Can you work these out from the model? Positions are in its coordinate system, mm. A direction names the side the tool comes from. Give positions to 0.01 mm unless a question says otherwise; leave off trailing zeros. Order: outer loops, then holes, each group sorted by start corner. A loop starts at its lowest first (then second) coordinate and runs counter-clockwise, first axis right, second up.
```python
from build123d import *

# Parameters (mm, degrees)
F0_W     = 127
F0_H     = 177.8
F1_DEPTH = 2.54
F2_W     = 127
F2_H     = 25.4
F3_DEPTH = 127
F4_W     = 25.4
F4_H     = 6.849984
F4_H_2   = 6.360701
F5_DEPTH = 7.62


with BuildPart() as f1:
    # F0 (on Top) → F1 (new body)
    with BuildSketch(Plane.XY):
        Rectangle(F0_W, F0_H)
    extrude(amount=-F1_DEPTH)

    # F2 (on face) → F3 (join)
    with BuildSketch(Plane.XY):
        with Locations((0, 76.2)):
            Rectangle(F2_W, F2_H)
    extrude(amount=F3_DEPTH)

    # F4 (on face) → F5 (join)
    with BuildSketch(Plane.XZ.offset(-63.5)):
        with Locations((-25.4, 42.159992)):
            Rectangle(F4_W, F4_H)
        with Locations((25.4, 41.915351)):
            Rectangle(F4_W, F4_H_2)
    extrude(amount=F5_DEPTH)


solid = f1.part
```
1) Suppose I cut it at A-A (x = -25). Please give me the cut outline in (y, z) (3 decimals).
2) Suppose I cut it at B-B (y = -74). Please give me the cut outline in (x, z), and give its area (3 significant figures).
3) I'm going to push flat-ended pins straight in: pin 1 Ø1.9 at (y, z) = (61.5, 43.5) entering from +X; pin 2 Ø6 at (x, y) = (-20, 58) entering from +Z (3 decimals); pin 3 Ø7 at (x, z) = (24, 43) entering from -Y. Where does each tip first touch, or does it pass through?
4) Suppose I cut it at C-C (z = 84). Please give me the cut outline in (x, y), and give its area (3 significant figures).
5) Suppose I cut it at D-D (x = 29). Please give me the cut outline in (y, z) (3 decimals), and give its area (3 significant figures).
6) Which directions (+Z, -Z, +X, -X, +Y, -Y) give clear straight access to the entire face, cutting with the end or side of a thin tool? Please do faces 5 (the face through (38.1, 60, 42)), 6 (the face through (-26, 60, 45.585)), 7 (the face through (-12.7, 60, 42)), 8 (the face through (-38.1, 60, 42)).
7) We'd pull the mould along Z, two halves only. Please class faces 1 (the face through (25, 60, 38.735)), 2 (the face through (25, 55.88, 42)), 3 (the face through (25, 60, 45.096)), 4 (the face through (-26, 60, 38.735)): +Z half, -Z half, draft (parallel to the pull), parting line (faces both ways), or undercut.
8) If I drill on line 1 (Z direction, x = 14.5, y = 60) (3 decimals); line 2 (Y direction, x = 17, z = 117); line 3 (Z direction, x = 38.5, y = 7), over which ranges is the centre line in solid material (lowest first)?
Results:
1. outline: (-88.9, -2.54) - (88.9, -2.54) - (88.9, 127) - (63.5, 127) - (63.5, 45.585) - (55.88, 45.585) - (55.88, 38.735) - (63.5, 38.735) - (63.5, 0) - (-88.9, 0) - close
2. outline: (-63.5, -2.54) - (63.5, -2.54) - (63.5, 0) - (-63.5, 0) - close
2. area: 323 mm2
3. pin 1: stops at x = 38.1
3. pin 2: stops at z = 45.585
3. pin 3: stops at y = 55.88
4. outline: (-63.5, 63.5) - (63.5, 63.5) - (63.5, 88.9) - (-63.5, 88.9) - close
4. area: 3,230 mm2
5. outline: (-88.9, -2.54) - (88.9, -2.54) - (88.9, 127) - (63.5, 127) - (63.5, 45.096) - (55.88, 45.096) - (55.88, 38.735) - (63.5, 38.735) - (63.5, 0) - (-88.9, 0) - close
5. area: 3,730 mm2
6. face 5: +Z, +X, -Y
6. face 6: +Z, +X, -X, -Y
6. face 7: +Z, -Y
6. face 8: +Z, -X, -Y
7. face 1: undercut
7. face 2: draft
7. face 3: +Z half
7. face 4: undercut
8. line 1: z = -2.54 to 0, 38.735 to 45.096
8. line 2: y = 63.5 to 88.9
8. line 3: z = -2.54 to 0
